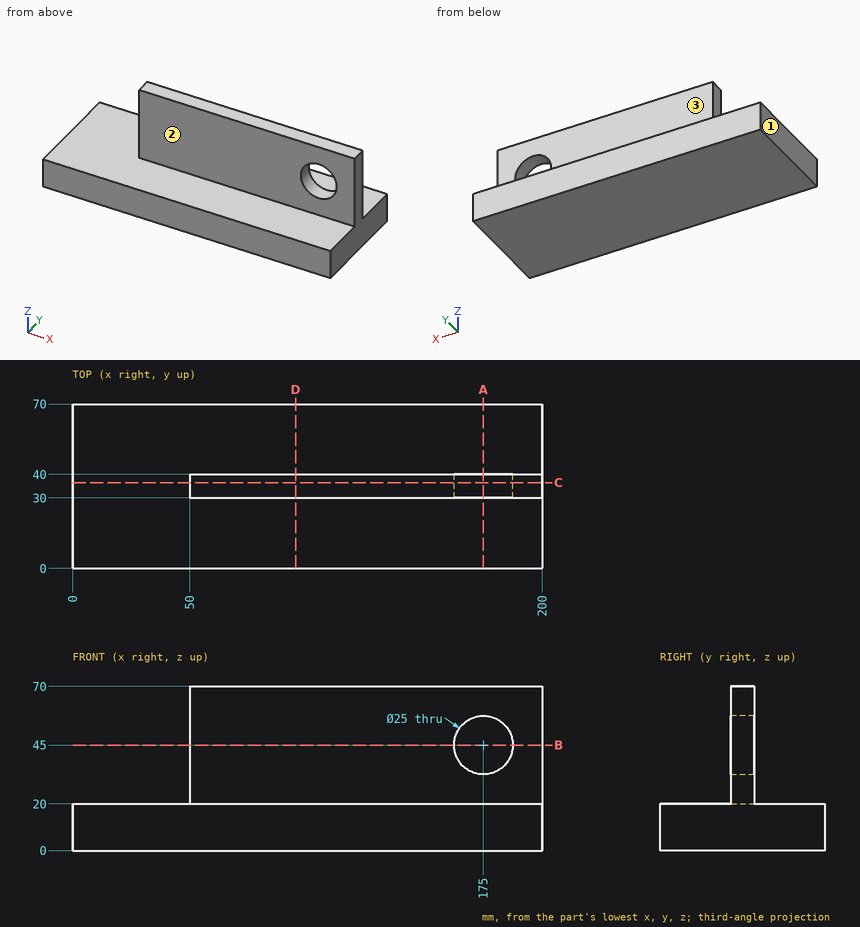
The figure shows three views and two pictorial views of one solid part (mm, origin at its lowest corner). Answer the questions. A direction names the side the tool comes from. Round coordinates to 2 decimals unless told otherwise and drop trailing zeros. Loops run counter-clockwise (first coordinate to the right, second up) from the corner with the lowest first, then second, coordinate; pieces in that order, holes last. Notation, with made-up numbers: (49, -6.5) - (107, -6.5) arc R14 ccw to (107, 17.5) - close; hole circle Ø11 at (-6.5, 25). An arc over 180 degrees is marked (long way). Use one line per item in the form item = value. Start each with the question number.
(1) Flat-ended cylindrical pins translate along their axes: P1, Ø2, axis at x = 113.5, y = 19.5, coming from the +Z side; P2, Ø20, axis at x = 175, z = 45, coming from the +Y side; P3, Ø1, axis at y = 33.5, z = 27, coming from the -X side; P4, Ø4, axis at x = 141.5, z = 61, coming from the +Y side. Find the tip coordinate at first contact, or state that the pin passes through.
(2) Consider line 1 (X direction, y = 36.25, z = 45); line 2 (Z direction, x = 140, y = 61.5); line 3 (Y direction, x = 103, z = 48). Determine where each line is inside the solid, lowest interval first.
(3) Which of the six approach directions +Z, -Z, +X, -X, +Y, -Y give full straight-line access (tool end or side, diameter ignored) to the marked faces 1, 2 and 3?
(4) Find section B-B on z = 45. Determine the outline of the cut face in (x, y), and give its area (3 significant figures).
(5) Find section A-A on x = 175. Determine the outline of the cut face in (y, z).
(6) Find section D-D on x = 95. Determine the outline of the cut face in (y, z), and give its area (3 significant figures).
(7) Find section C-C on y = 36.5. Determine the outline of the cut face in (x, z).
Answer list:
q1.P1 = 20
q1.P2 = through
q1.P3 = 50
q1.P4 = 40
q2.line_1 = 50 to 162.5, 187.5 to 200
q2.line_2 = 0 to 20
q2.line_3 = 30 to 40
q3.face_1 = +Z, -Z, -X, +Y, -Y
q3.face_2 = +Z, +X, -X, -Y
q3.face_3 = +Z, +X, -X, +Y
q4.outline = (50, 30) - (162.5, 30) - (162.5, 40) - (50, 40) - close; (187.5, 30) - (200, 30) - (200, 40) - (187.5, 40) - close
q4.area = 1,250 mm^2
q5.outline = (0, 0) - (70, 0) - (70, 20) - (40, 20) - (40, 32.5) - (30, 32.5) - (30, 20) - (0, 20) - close; (30, 57.5) - (40, 57.5) - (40, 70) - (30, 70) - close
q6.outline = (0, 0) - (70, 0) - (70, 20) - (40, 20) - (40, 70) - (30, 70) - (30, 20) - (0, 20) - close
q6.area = 1,900 mm^2
q7.outline = (0, 0) - (200, 0) - (200, 70) - (50, 70) - (50, 20) - (0, 20) - close; hole circle Ø25 at (175, 45)
